```python
from build123d import *

# Parameters (mm, degrees)
SKETCH1_W           = 47.5
SKETCH1_H           = 27
SKETCH1_W_2         = 41.5
SKETCH1_H_2         = 21
BOSS_EXTRUDE2_DEPTH = 30
SKETCH2_W           = 9.308114218
SKETCH2_H           = 23.373709037
CUT_EXTRUDE1_DEPTH  = 30
SKETCH3_W           = 25.956751415
SKETCH3_H           = 3
BOSS_EXTRUDE3_DEPTH = 8
SKETCH4_W           = 27
SKETCH4_H           = 3
BOSS_EXTRUDE4_DEPTH = 8
SKETCH5_R           = 14.75
SKETCH5_R_2         = 12.75
BOSS_EXTRUDE5_DEPTH = 25


with BuildPart() as part:
    # Sketch1 → Boss-Extrude2 (new body)
    with BuildSketch(Plane(origin=(0, 0, 0), x_dir=(1, 0, 0), z_dir=(0, 1, 0))):
        with Locations((34.749341264, 5.949225985)):
            Rectangle(SKETCH1_W, SKETCH1_H)
        with Locations((34.749341264, 5.949225985)):
            Rectangle(SKETCH1_W_2, SKETCH1_H_2, mode=Mode.SUBTRACT)
    extrude(amount=-BOSS_EXTRUDE2_DEPTH)

    # Sketch2 → Cut-Extrude1 (cut)
    with BuildSketch(Plane.ZY.offset(-10.999341264)):
        with Locations((-6.259496459, -16.501916984)):
            Rectangle(SKETCH2_W, SKETCH2_H)
    extrude(amount=-CUT_EXTRUDE1_DEPTH, mode=Mode.SUBTRACT)

    # Sketch3 → Boss-Extrude3 (add)
    with BuildSketch(Plane.ZY.offset(-10.999341264)):
        with Locations((-6.067211219, -1.5)):
            Rectangle(SKETCH3_W, SKETCH3_H)
    extrude(amount=BOSS_EXTRUDE3_DEPTH)

    # Sketch4 → Boss-Extrude4 (add)
    with BuildSketch(Plane(origin=(58.499341264, 0, 0), x_dir=(0, 0, -1), z_dir=(1, 0, 0))):
        with Locations((5.949225985, -1.5)):
            Rectangle(SKETCH4_W, SKETCH4_H)
    extrude(amount=BOSS_EXTRUDE4_DEPTH)

    # Sketch5 → Boss-Extrude5 (add)
    with BuildSketch(Plane(origin=(0, 0, -19.449225985), x_dir=(-1, 0, 0), z_dir=(0, 0, -1))):
        with Locations(Location((-25.775893869, -15, 0), (0, 0, 180))):
            Circle(SKETCH5_R)
        with Locations((-25.775893869, -15)):
            Circle(SKETCH5_R_2, mode=Mode.SUBTRACT)
    extrude(amount=BOSS_EXTRUDE5_DEPTH)


solid = part.part
```
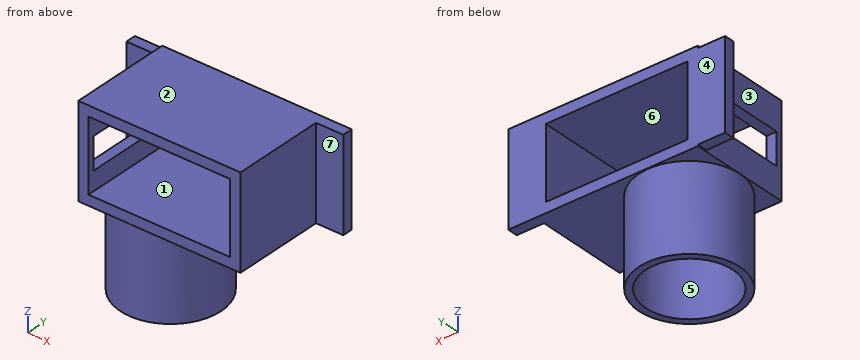
The model under review builds one solid part; all positions refer to its coordinate system, in mm. Face numbers are marked on the shaded views. A direction names the side the tool comes from. Give positions to 0.01 mm unless a question says otherwise; leave off trailing zeros. Order: outer loops, then holes, each group sorted by start corner. A loop starts at its lowest first (then second) coordinate and runs counter-clockwise, first axis right, second up. Notation, with made-up numbers: (-21.5, 13.5) - (27.5, 13.5) arc R11 ccw to (27.5, 34.5) - close; hole circle Ø3 at (29, -11.5). An arc over 180 degrees is marked (long way). Use CSV: the item, a comma, the result in double quotes. Start each with the question number.
Q1. To check wall thickness, follow line 1 along X through (y, z) = (-4, -14.5); line 2 along Z through (x, y) = (31, -13.5); line 3 along X through (y, z) = (-14.75, -37). State the ranges of each line that lie inside material, in increasing order. Write a range as [from, to].
Q2. We need section A-A, the plane z = 3.5. Write out the cut boundary in (x, y), and give its area (3 significant figures).
Q3. Tool access review of the marked faces 4, 5, 6 and 7: name each direction out of +Z, -Z, +X, -X, +Y, -Y from which nothing blocks a thin tool from reaching the whole face with its end or side.
Q4. The part is to be moulded in two halves that separate along Z. For the marked faces 1, 2 and 3, say which applies: +Z half, -Z half, draft (parallel to the pull), parting line (faces both ways), or undercut.
Q5. Clearance check with flat-ended pins moving along their axes: pin 1 Ø1.5 at (x, z) = (31.5, -22.5) entering from -Y; pin 2 Ø5 at (x, y) = (46.5, -6.5) entering from -Z; pin 3 Ø6.5 at (y, z) = (-13, -5.5) entering from +X; pin 4 Ø4 at (x, z) = (27, -15) entering from -Y. State where each tip first meets the part, or that it passes through.
Q6. We need section B-B, the plane x = 46.5. Write out the cut boundary in (y, z).
Q7. We need section C-C, the plane z = -5.5. Write out the cut boundary in (x, y), and give its area (3 significant figures).
Outcome:
1,line 1,"x = [11, 14], [55.5, 58.5]"
1,line 2,"z = [-19.45, -16.45], [4.55, 7.55]"
1,line 3,"x = [11.03, 13.03], [38.52, 40.52]"
2,outline,"(3, -3) - (11, -3) - (11, -30) - (14, -30) - (14, 0) - (3, 0) - close; (55.5, -30) - (58.5, -30) - (58.5, -3) - (66.5, -3) - (66.5, 0) - (55.5, 0) - close"
2,area,"228 mm^2"
3,face 4,"+Z, -Z, +X, -X, +Y"
3,face 5,"-Z"
3,face 6,"+Y, -Y"
3,face 7,"+Z, -Z, +X, -Y"
4,face 1,"undercut"
4,face 2,"+Z half"
4,face 3,"draft"
5,pin 1,"stops at y = -28.89"
5,pin 2,"stops at z = -19.45"
5,pin 3,"stops at x = 58.5"
5,pin 4,"stops at y = -30"
6,outline,"(-30, -19.45) - (0, -19.45) - (0, -16.45) - (-30, -16.45) - close; (-30, 4.55) - (0, 4.55) - (0, 7.55) - (-30, 7.55) - close"
7,outline,"(3, -3) - (11, -3) - (11, -4.82) - (14, -4.82) - (14, 0) - (3, 0) - close; (11, -30) - (14, -30) - (14, -28.19) - (11, -28.19) - close; (55.5, -30) - (58.5, -30) - (58.5, -3) - (66.5, -3) - (66.5, 0) - (55.5, 0) - close"
7,area,"158 mm^2"
